Here's the drawing with two shaded views (mm, measured from the low corner). I have some questions. A direction names the side the tool comes from. Coordinates: 2 decimals unless noted, no trailing zeros. Write each loop counter-clockwise with the first axis right and the second up, starting at its lowest first coordinate (ties: lowest second). Pieces come first, ordered by that corner, then holes. Notation, with made-up numbers: (-1.75, -26) -> (44.25, -26) arc R22 cw to (44.25, -12) -> close; hole circle Ø5 at (-32, 19). An arc over 180 degrees is marked (long way). Answer in a Markdown table with one row per item. Add a question column.
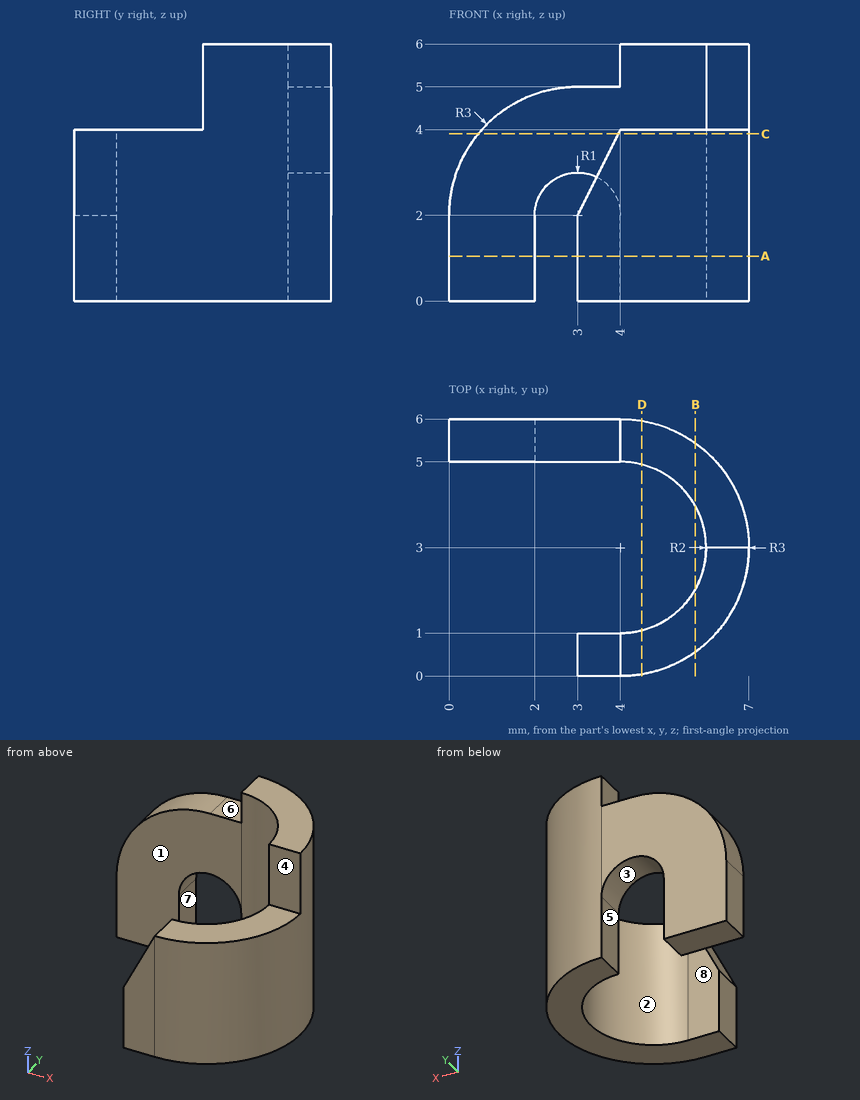
Q1. Imagine slicing it at B-B on x = 5.75. Please give me the cut outline in (y, z), plus the area to 3 significant figures.
Q2. Imagine slicing it at C-C on z = 3.9. Please give me the cut outline in (x, y), plus the area to 3 significant figures.
Q3. I need wall thicknesses on line 1 (Y direction, x = 2.25, z = 3.6); line 2 (Y direction, x = 4.5, z = 1); line 3 (X direction, y = 3.05, z = 1.7). Which ranges of each line are inside material? Lowest first, please. Write a range as [from, to].
Q4. Imagine slicing it at D-D on x = 4.5. Please give me the cut outline in (y, z).
Q5. For the marked faces 4, 5, 6, 7 and 8, which set-ups out of +Z, -Z, +X, -X, +Y, -Y let a thin tool reach every point of the face, with its end or its side?
Q6. If we mould it in two halves opening along X, with no side actions, what happens to the marked faces 1, 2 and 3? For each: pulls with the +X half, pulls with the -X half, needs draft (parallel to the pull), parting line crosses it, or undercut.
Q7. Imagine slicing it at A-A on z = 1.05. Please give me the cut outline in (x, y).
Q8. I'm going to push flat-ended pins straight in: P1, Ø0.8, axis at y = 0.5, z = 0.5, coming from the -X side; P2, Ø0.8, axis at x = 6.5, z = 5, coming from the -Y side; P3, Ø0.8, axis at y = 5.5, z = 5.5, coming from the -X side. Where does each tip first touch, or does it pass through?
Result sheet:
| question | item | result |
|---|---|---|
| 1 | outline | (0.56, 0) -> (2.03, 0) -> (2.03, 4) -> (0.56, 4) -> close; (3.97, 0) -> (5.44, 0) -> (5.44, 6) -> (3.97, 6) -> close |
| 1 | area | 14.7 mm^2 |
| 2 | outline | (0.68, 5) -> (4, 5) arc R2 cw to (4, 1) -> (3.95, 1) -> (3.95, 0) -> (4, 0) arc R3 ccw to (4, 6) -> (0.68, 6) -> close |
| 2 | area | 11.2 mm^2 |
| 3 | line 1 | y = [5, 6] |
| 3 | line 2 | y = [0.04, 1.06], [4.94, 5.96] |
| 3 | line 3 | x = [6, 7] |
| 4 | outline | (0.04, 0) -> (1.06, 0) -> (1.06, 4) -> (0.04, 4) -> close; (4.94, 0) -> (5.96, 0) -> (5.96, 6) -> (4.94, 6) -> close |
| 5 | face 4 | +Z, +X, -X, -Y |
| 5 | face 5 | -Z, +Y |
| 5 | face 6 | +Z, -X, +Y, -Y |
| 5 | face 7 | -Z, +Y, -Y |
| 5 | face 8 | +Z, -Z, -X |
| 6 | face 1 | needs draft |
| 6 | face 2 | pulls with the -X half |
| 6 | face 3 | undercut |
| 7 | outline | (0, 5) -> (2, 5) -> (2, 6) -> (0, 6) -> close; (3, 0) -> (4, 0) arc R3 ccw to (4, 6) -> (4, 5) arc R2 cw to (4, 1) -> (3, 1) -> close |
| 8 | P1 | stops at x = 3 |
| 8 | P2 | stops at y = 3 |
| 8 | P3 | stops at x = 4 |
